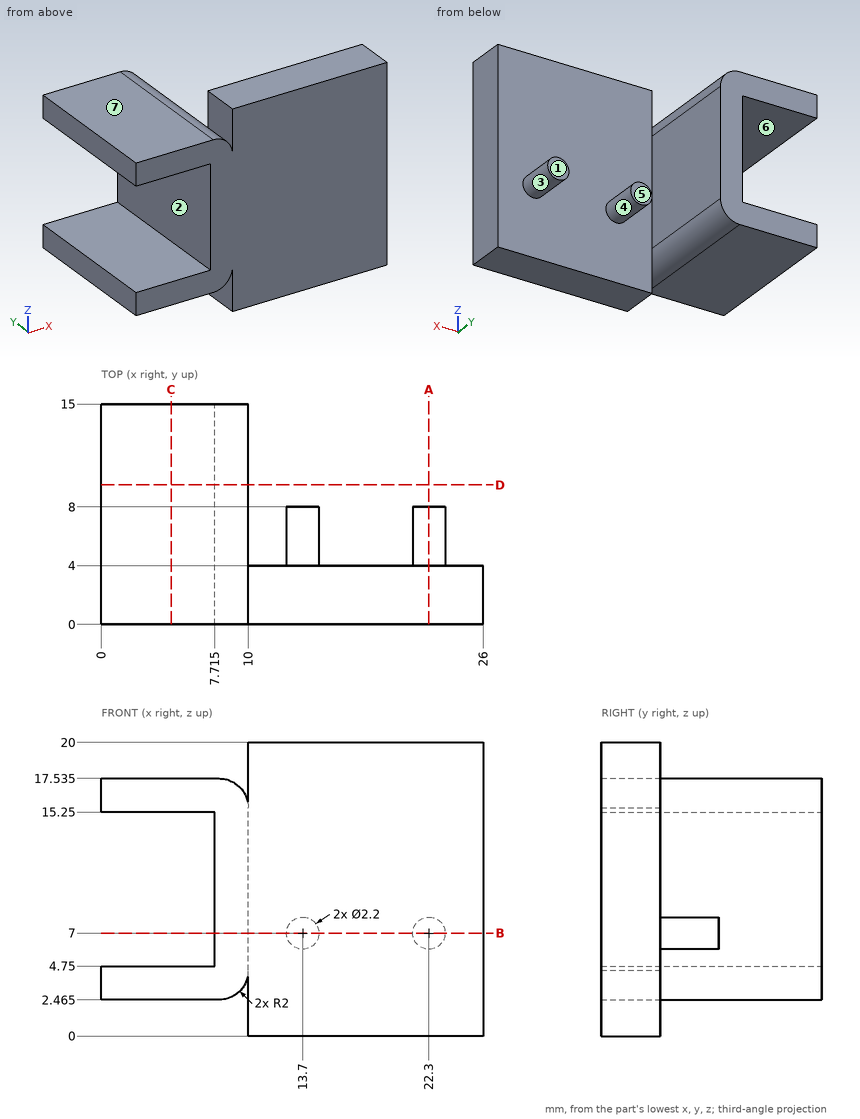
Verification items for this drawing (mm, ordinates from the low corner). A direction names the side the tool comes from. Coordinates: 2 decimals unless noted, no trailing zeros. Order: outer loops, then holes, each group sorted by start corner. A loop starts at its lowest first (then second) coordinate and runs counter-clockwise, first axis right, second up. Notation, with made-up numbers: M -1.5,74 L 27.5,74 A14 ccw 27.5,78 Z; hole C -18.5,72 d1. An arc over 180 degrees is marked long. One line per item, written item: value. Start each with the question number.
Item 1: Sectioned sample at B-B on z = 7. Record the cut outline in (x, y) (3 decimals), then the cut area to 3 significant figures.
Item 2: Sectioned sample at C-C on x = 4.75. Record the cut outline in (y, z) (3 decimals), then the cut area to 4 significant figures.
Item 3: Mould release check, pull along X, two halves, no side actions. Record for the marked faces 1, 2 and 3: pulls with the +X half, pulls with the -X half, needs draft (parallel to the pull), parting line crosses it, or undercut.
Item 4: Depth check by flat-ended pin: P1, Ø8.5, axis at x = 3.5, y = 7.5, coming from the +Z side (3 decimals); P2, Ø9, axis at x = 5.5, y = 9, coming from the -Z side (3 decimals); P3, Ø1.5, axis at y = 8.5, z = 4.5, coming from the +X side. Enter the tip coordinate at first touch or a pass-through.
Item 5: Sectioned sample at A-A on x = 22.3. Record the cut outline in (y, z).
Item 6: Access from +Z, -Z, +X, -X, +Y, -Y to the whole of each face (thin tool, end or side, straight path). Record for the marked faces 4, 5, 6 and 7.
Item 7: Thickness scan on probe 1 along Z at (x, y) = (2.5, 5) (3 decimals); probe 2 along X at (y, z) = (2.75, 13.25) (3 decimals); probe 3 along Y at (x, z) = (16, 7.75). Record the ranges inside material, lowest first.
Item 8: Sectioned sample at D-D on y = 9.5. Record the cut outline in (x, z) (3 decimals), then the cut area to 3 significant figures.
Calculated:
1. outline: M 7.715,0 L 26,0 L 26,4 L 23.4,4 L 23.4,8 L 21.2,8 L 21.2,4 L 14.8,4 L 14.8,8 L 12.6,8 L 12.6,4 L 10,4 L 10,15 L 7.715,15 Z
1. area: 116 mm^2
2. outline: M 0,2.465 L 15,2.465 L 15,4.75 L 0,4.75 Z; M 0,15.25 L 15,15.25 L 15,17.535 L 0,17.535 Z
2. area: 68.55 mm^2
3. face 1: needs draft
3. face 2: pulls with the -X half
3. face 3: undercut
4. P1: z = 17.535
4. P2: z = 2.465
4. P3: x = 10
5. outline: M 0,0 L 4,0 L 4,5.9 L 8,5.9 L 8,8.1 L 4,8.1 L 4,20 L 0,20 Z
6. face 4: +Y
6. face 5: +Z, -Z, +X, +Y
6. face 6: -X, +Y, -Y
6. face 7: +Z, -X, +Y, -Y
7. probe 1: 2.465 to 4.75, 15.25 to 17.535
7. probe 2: 7.715 to 26
7. probe 3: 0 to 4
8. outline: M 0,2.465 L 8,2.465 A2 ccw 10,4.465 L 10,15.535 A2 ccw 8,17.535 L 0,17.535 L 0,15.25 L 7.715,15.25 L 7.715,4.75 L 0,4.75 Z
8. area: 68.0 mm^2
